Here's the drawing with two shaded views (mm, measured from the low corner). I have some questions. A direction names the side the tool comes from. Give positions to 0.01 mm unless a question says otherwise; leave off trailing zeros. Loops run counter-clockwise (first coordinate to the right, second up) from the corner with the lowest first, then second, coordinate; pieces in that order, holes last. Notation, with made-up numbers: (21, -1) -> (74, -1) arc R18 ccw to (74, 21) -> close; hole circle Ø5 at (26, 86.25). An arc over 180 degrees is marked (long way). Answer in a Markdown table with one row per item. Add a question column.
Item 1: If I drill on line 1 (Z direction, x = 5.5, y = 6.5); line 2 (Y direction, x = 12.25, z = 24.5); line 3 (Y direction, x = 15.75, z = 23), over which ranges is the centre line in solid material (lowest first)?
Item 2: Which directions (+Z, -Z, +X, -X, +Y, -Y) give clear straight access to the entire face, cutting with the end or side of a thin tool? Please do the marked faces 1 and 2.
Item 3: If we section it at C-C (z = 14): Write out the boundary of the cut face in (x, y), then the cut area to 3 significant figures.
Item 4: If we section it at D-D (z = 33.5): Write out the boundary of the cut face in (x, y).
Item 5: For P1, Ø6, axis at x = 6.5, y = 19, coming from the +Z side; P2, Ø1, axis at y = 7.5, z = 9.5, coming from the +X side; P3, Ø2, axis at y = 14.5, z = 23.5, coming from the -X side, each with a flat end and sliding along its axis, tell me the tip position at first contact or that it passes through.
Item 6: If we section it at A-A (x = 12): Write out the boundary of the cut face in (y, z), then the cut area to 3 significant figures.
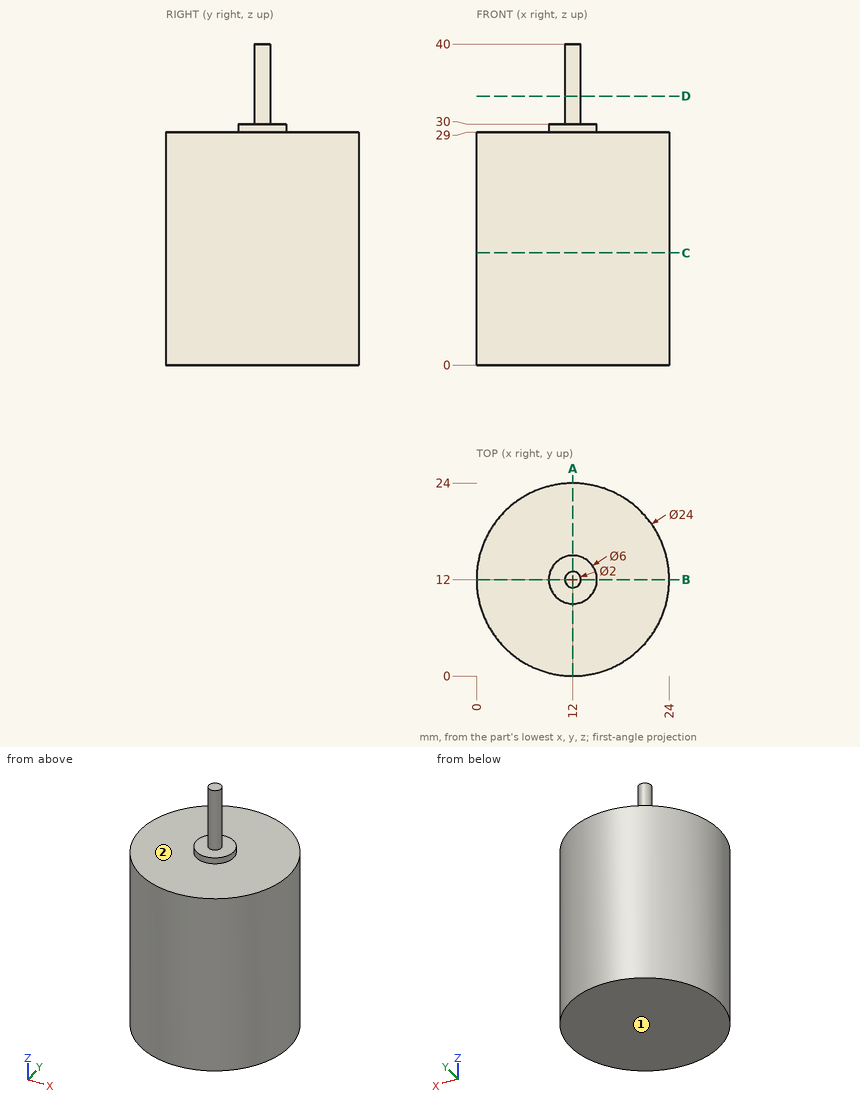
Recorded:
| question | item | result |
|---|---|---|
| 1 | line 1 | z = 0 to 29 |
| 1 | line 2 | y = 0 to 24 |
| 1 | line 3 | y = 0.6 to 23.4 |
| 2 | face 1 | -Z, +X, -X, +Y, -Y |
| 2 | face 2 | +Z |
| 3 | outline | circle Ø24 at (12, 12) |
| 3 | area | 452 mm^2 |
| 4 | outline | circle Ø2 at (12, 12) |
| 5 | P1 | stops at z = 29 |
| 5 | P2 | stops at x = 23.31 |
| 5 | P3 | stops at x = 0.09 |
| 6 | outline | (0, 0) -> (24, 0) -> (24, 29) -> (15, 29) -> (15, 30) -> (13, 30) -> (13, 40) -> (11, 40) -> (11, 30) -> (9, 30) -> (9, 29) -> (0, 29) -> close |
| 6 | area | 722 mm^2 |
